Read the model definition and answer for the solid it produces. Units are mm, in the model's axes. A direction names the side the tool comes from. Round coordinates to 2 decimals unless told otherwise and drop trailing zeros. Loops run counter-clockwise (first coordinate to the right, second up) from the corner with the lowest first, then second, coordinate; pieces in that order, holes last. Notation, with made-up numbers: M -19,31 L -14,31 A28 ccw -14,67 Z; hole C -25,85 d8. An arc over 180 degrees is marked long. Write each question's results on one line, items separated by ' | '.
from build123d import *

# Parameters (mm, degrees)
SKETCH2_R           = 48
BOSS_EXTRUDE1_DEPTH = 4
BOSS_EXTRUDE2_DEPTH = 14
SKETCH31_R          = 6.5
CUT_EXTRUDE18_DEPTH = 96.977067922
CUT_EXTRUDE19_DEPTH = 10
SKETCH32_R          = 1
CUT_EXTRUDE20_DEPTH = 4.5
SKETCH33_R          = 43.5
BOSS_EXTRUDE3_DEPTH = 2.2
SKETCH35_R          = 7
CUT_EXTRUDE22_DEPTH = 93.968532394
SKETCH36_R          = 2.701818283
CUT_EXTRUDE24_DEPTH = 86.072189458
SKETCH37_R          = 1
CUT_EXTRUDE25_DEPTH = 4.5


with BuildPart() as part:
    # Sketch2 → Boss-Extrude1 (new body)
    with BuildSketch(Plane(origin=(0, 0, 0), x_dir=(1, 0, 0), z_dir=(0, 1, 0))):
        with Locations(Location((0, 0, 0), (0, 0, 270))):
            Circle(SKETCH2_R)
    extrude(amount=BOSS_EXTRUDE1_DEPTH)

    # Sketch7 → Boss-Extrude2 (add)
    with BuildSketch(Plane(origin=(-4, 0, 0), x_dir=(0, 0, -1), z_dir=(1, 0, 0))):
        with BuildLine():
            Line((18.652115716, 4), (18.652115716, 16.356133126))
            ThreePointArc((18.652115716, 16.356133126), (20.111216245, 23.455333411), (24.251965127, 29.403595153))
            ThreePointArc((24.251965127, 29.403595153), (24.659117989, 50.747356958), (3.311904584, 50.883081894))
            Line((3.311904584, 50.883081894), (-22.631121669, 24.94005564))
            ThreePointArc((-22.631121669, 24.94005564), (-28.050440452, 16.82947192), (-29.95345214, 7.262386111))
            Line((-29.95345214, 7.262386111), (-29.95345214, 4))
            Line((-29.95345214, 4), (18.652115716, 4))
        make_face()
    extrude(amount=-BOSS_EXTRUDE2_DEPTH)

    # Sketch31 → Cut-Extrude18 (cut, through all)
    with BuildSketch(Plane(origin=(-18, 10.461755651, -5.359516796), x_dir=(0, 0, 1), z_dir=(-1, 0, 0))):
        with Locations((-4.922469695, 24.905412087)):
            Circle(SKETCH31_R)
    extrude(amount=-CUT_EXTRUDE18_DEPTH, mode=Mode.SUBTRACT)

    # Sketch31_3 → Cut-Extrude19 (cut)
    with BuildSketch(Plane(origin=(-18, 10.461755651, -5.359516796), x_dir=(0, 0, 1), z_dir=(-1, 0, 0))):
        Polygon((-5.41546104, 34.054639751), (11.74960782, 18.74580534), (3.09678837, 9.043809897), (-14.06828049, 24.352644308), align=None)
    extrude(amount=-CUT_EXTRUDE19_DEPTH, mode=Mode.SUBTRACT)

    # Sketch32 → Cut-Extrude20 (cut)
    with BuildSketch(Plane.ZY.offset(18)):
        with Locations((-17.080620038, 41.264504586)):
            Circle(SKETCH32_R)
        with Locations((3.929449654, 22.692559529)):
            Circle(SKETCH32_R)
    extrude(amount=-CUT_EXTRUDE20_DEPTH, mode=Mode.SUBTRACT)

    # Sketch33 → Boss-Extrude3 (add)
    with BuildSketch(Plane.XZ):
        with Locations(Location((0, 0, 0), (0, 0, 270))):
            Circle(SKETCH33_R)
    extrude(amount=BOSS_EXTRUDE3_DEPTH)

    # Sketch35 → Cut-Extrude22 (cut, through all)
    with BuildSketch(Plane(origin=(-3.192833023, 4, -10.250875044), x_dir=(1, 0, 0), z_dir=(0, 1, 0))):
        with Locations(Location((7.665516898, 0, 0), (0, 0, 270))):
            Circle(SKETCH35_R)
    extrude(amount=-CUT_EXTRUDE22_DEPTH, mode=Mode.SUBTRACT)

    # Sketch36 → Cut-Extrude24 (cut, through all)
    with BuildSketch(Plane(origin=(0, 4, 0), x_dir=(1, 0, 0), z_dir=(0, 1, 0))):
        with Locations((2.310071728, 4.444115209)):
            Circle(SKETCH36_R)
    extrude(amount=-CUT_EXTRUDE24_DEPTH, mode=Mode.SUBTRACT)

    # Sketch37 → Cut-Extrude25 (cut)
    with BuildSketch(Plane(origin=(0, 4, 0), x_dir=(1, 0, 0), z_dir=(0, 1, 0))):
        with Locations(Location((4.472683875, 19.750875044, 0), (0, 0, 270))):
            Circle(SKETCH37_R)
    extrude(amount=-CUT_EXTRUDE25_DEPTH, mode=Mode.SUBTRACT)


solid = part.part
Item 1: The part is cut by section C-C (x = -31). Determine the outline of the cut face in (y, z).
Outcome:
outline: M -2.2,-30.52 L 0,-30.52 L 0,-36.65 L 4,-36.65 L 4,36.65 L 0,36.65 L 0,30.52 L -2.2,30.52 Z
Item 2: The part is cut by section B-B (z = 0). Determine the outline of the cut face in (x, y).
Outcome:
outline: M -48,0 L -43.5,0 L -43.5,-2.2 L 43.5,-2.2 L 43.5,0 L 48,0 L 48,4 L -4,4 L -4,47.57 L -18,47.57 L -18,34.91 L -8,34.91 L -8,22.04 L -18,22.04 L -18,4 L -48,4 Z
Item 3: The part is cut by section A-A (y = 37). Determine the outline of the cut face in (x, z), plus the area to 3 significant figures.
Outcome:
outline: M -18,-28.56 L -4,-28.56 L -4,-16.57 L -8,-16.57 L -8,-17.48 L -18,-17.48 Z; M -18,-2.35 L -8,-2.35 L -8,-3.99 L -4,-3.99 L -4,10.57 L -18,10.57 Z | area: 346 mm2
Item 4: For faces 4 (the face through (-18, 19, 1)), 5 (the face through (-13.07, 42.337, -12.719)), 6 (the face through (-7.987, 39.76, -15.073)), 7 (the face through (-11, 10, -18.652)), 8 (the face through (14.418, 1.972, 45.783)), determine the directions among +Z, -Z, +X, -X, +Y, -Y from which every point of the face is accessible in a straight line to the end or side of a thin tool.
Outcome:
face 4: +Z, -Z, -X, +Y | face 5: -X | face 6: +X, -X | face 7: -Z, +X, -X | face 8: +Y, -Y
Item 5: Straight lines are drawn through the part: line 1 (Y direction, x = 4, z = -2); line 2 (X direction, y = 7.5, z = 25); line 3 (Y direction, x = 18.5, z = -43.5). For each, find the intervals that lie inside material, in ascending order.
Outcome:
line 1: y = -2.2 to 4 | line 2: x = -18 to -4 | line 3: y = 0 to 4
Item 6: The part is cut by section D-D (y = 2.5). Determine the outline of the cut face in (x, z), plus the area to 3 significant figures.
Outcome:
outline: C 0,0 d96; hole M -0.3,-5.13 A7 ccw long 4.74,-3.26 A2.7 ccw Z; hole C 4.47,-19.75 d2 | area: 7,070 mm2
Item 7: Flat-ended cylindrical pins translate along their axes: pin 1 (10 mm diameter, centred on x = -12, y = 12.5, fed in from -Z); pin 2 (1.5 mm diameter, centred on y = 26, z = 24, fed in from -X); pin 3 (1.8 mm diameter, centred on y = 22.69, z = 3.93, fed in from +X); pin 4 (15.5 mm diameter, centred on y = 24, z = 14.5, fed in from -X). Find the tip coordinate at first contact, or state that the pin passes through.
Outcome:
pin 1: stops at z = -18.69 | pin 2: passes through | pin 3: stops at x = -4 | pin 4: stops at x = -18
Item 8: The mould has two halves that part along Z. Classify faces 1 (the face through (-13.07, 36.969, -2.313)), 2 (the face through (-4, 24, 1)), 3 (the face through (-10.9, 23.36, -20.07)): pulls with the +Z half, pulls with the -Z half, needs draft (parallel to the pull), parting line crosses it, or undercut.
Outcome:
face 1: undercut | face 2: needs draft | face 3: pulls with the -Z half
